Input: part model. Units: mm. Frame: model coordinates. A direction names the side the tool comes from. Round coordinates to 2 decimals unless told otherwise and drop trailing zeros. Order: outer loops, then holes, each group sorted by start corner. A loop starts at its lowest first (then second) coordinate and runs counter-clockwise, first axis right, second up. Notation, with made-up numbers: M 12,-26 L 21,-26 A20 cw 21,3 Z; hole C 82,67.25 d8. An arc over 180 degrees is marked long. One line per question, with ' | ' between items.
Autodesk Inventor part; units mm, degrees
ref_plane "YZ Plane" through (0, 0, 0) normal (1, 0, 0) x (0, 1, 0)
ref_plane "XZ Plane" through (0, 0, 0) normal (0, 1, 0) x (-1, 0, 0)
ref_plane "XY Plane" through (0, 0, 0) normal (0, 0, 1) x (1, 0, 0)
sketch "Sketch2" plane through (0, 0, 0) normal (0, 1, 0) x (-1, 0, 0)
  circle A0 centre (0, 0) radius 25
  dimension "d0" = 50
extrude "Extrusion1" add sketch "Sketch2" along normal blind 200
sketch "Sketch3" plane through (0, 0, 0) normal (0, -1, 0) x (1, 0, 0)
  circle A0 centre (0, 0) radius 10
  dimension "d3" = 20
extrude "Extrusion2" add sketch "Sketch3" along normal blind 30
fillet "Fillet1" radius 2 3 edges at (25, 0, 0) (-10, -30, 0) (-10, 0, 0)
fillet "Fillet2" radius 2 1 edges at (25, 200, 0)
properties part number "plasmatorch"
Item 1: Section query C-C, the plane y = 52. Return loops of the section in (x, z).
Report:
outline: C 0,0 d50
Item 2: Section query A-A, the plane z = 0. Return loops of the section in (x, y), plus the area to 3 significant figures.
Report:
outline: M -25,2 A2 ccw -23,0 L -12,0 A2 cw -10,-2 L -10,-28 A2 ccw -8,-30 L 8,-30 A2 ccw 10,-28 L 10,-2 A2 cw 12,0 L 23,0 A2 ccw 25,2 L 25,198 A2 ccw 23,200 L -23,200 A2 ccw -25,198 Z | area: 10,600 mm²
Item 3: Line query: line 1 along Y through (x, z) = (-1, 23); line 2 along X through (y, z) = (175, -1); line 3 along X through (y, z) = (107, -4.5). Output: solid intervals per line, ascending. Write a range as from..to.
Report:
line 1: 0..200 | line 2: -24.98..24.98 | line 3: -24.59..24.59
Item 4: Section query B-B, the plane x = 0. Return loops of the section in (y, z).
Report:
outline: M -30,-8 A2 ccw -28,-10 L -2,-10 A2 cw 0,-12 L 0,-23 A2 ccw 2,-25 L 198,-25 A2 ccw 200,-23 L 200,23 A2 ccw 198,25 L 2,25 A2 ccw 0,23 L 0,12 A2 cw -2,10 L -28,10 A2 ccw -30,8 Z
Item 5: First-contact query: pin 1 (12 mm diameter, centred on y = -3, z = -17.5, fed in from -X); pin 2 (5 mm diameter, centred on y = 83, z = 18.5, fed in from +X); pin 3 (1.5 mm diameter, centred on x = 19, y = 56.5, fed in from -Z). Flat tips, straight axial feed; report the tip coordinate or a pass-through.
Report:
pin 1: x = -21.03 | pin 2: x = 19.21 | pin 3: z = -17.09
Item 6: Access query for faces 1 (the cylindrical face through (-2.17, -14.82, 9.76)), 2 (the flat face through (0, -30, 0)). Directions: +Z, -Z, +X, -X, +Y, -Y. A direction counts if a zero-diameter tool reaches every point of the face in a straight line with its end or side. Return the directions, or none.
Report:
face 1: -Y | face 2: +Z, -Z, +X, -X, -Y
